Check sheet for the modelled part. Datum: model origin and axes. Units: mm. A direction names the side the tool comes from. Give positions to 0.01 mm unless a question says otherwise; leave off trailing zeros. Loops run counter-clockwise (first coordinate to the right, second up) from the corner with the lowest first, then second, coordinate; pieces in that order, holes last. Notation, with made-up numbers: (-18, 18.5) -> (-5, 18.5) arc R15 cw to (-5, 42.5) -> close; hole circle Ø10 at (-30, 89.25). An arc over 180 degrees is marked (long way). Answer as CSV lines item,"result". Start each with the question number.
(1) Gauge pin test, flat ends, axial feed: pin 1 Ø0.8 at (x, y) = (-133, 20) entering from +Z (3 decimals); pin 2 Ø9.5 at (x, y) = (15, 28.5) entering from -Z; pin 3 Ø1.3 at (y, z) = (12.5, -132.5) entering from +X (3 decimals). Record the tip position at first contact, or that the pin passes through.
(2) Access from +Z, -Z, +X, -X, +Y, -Y to the whole of each face (thin tool, end or side, straight path). Record for faces 5 (the face through (-59.797, 5.027, -62.042)), 6 (the face through (35, 19, -131.724)), 7 (the face through (-85.2, 18.46, -85.23)).
(3) Material ranges on line 1 (Y direction, x = -53, z = -52) (3 decimals); line 2 (X direction, y = 6, z = -23.5) (3 decimals); line 3 (Z direction, x = -102, y = 2) (3 decimals), recorded low to high. Write a range as from..to.
(4) Section check B-B on x = -49.5. Enter the section's corners in (y, z) (3 decimals), plus the area to 3 significant figures.
(5) Section check A-A on z = -82. Enter the section's corners in (x, y) (3 decimals), plus the area to 3 significant figures.
(6) Release check for a two-part mould opening along Y. For faces 1 (the face through (-97, 11.176, -89)), 2 (the face through (36.908, 6.437, -130.973)), 3 (the face through (-45, 0, -46)), 4 (the face through (0, 4, -86)) record: pulls with the +Y half, pulls with the -Y half, needs draft (parallel to the pull), parting line crosses it, or undercut.
(7) Section check C-C on z = -119. Enter the section's corners in (x, y) (3 decimals), plus the area to 3 significant figures.
from build123d import *

# Parameters (mm, degrees)
SKETCH1_R            = 15
BOSS_EXTRUDE2_DEPTH  = 8.255
BOSS_EXTRUDE3_DEPTH  = 8.255
BOSS_EXTRUDE4_DEPTH  = 38.1
SKETCH5_R            = 3.249999977
CUT_EXTRUDE3_DEPTH   = 63.5
BOSS_EXTRUDE9_DEPTH  = 3.175
BOSS_EXTRUDE11_DEPTH = 3.175
BOSS_EXTRUDE14_DEPTH = 3.175
SKETCH15_W           = 38.1
SKETCH15_H           = 44.45
BOSS_EXTRUDE15_DEPTH = 1.524
SKETCH16_W           = 38.1
SKETCH16_H           = 44.45
BOSS_EXTRUDE16_DEPTH = 1.524
SKETCH17_R           = 1.98501
CUT_EXTRUDE4_DEPTH   = 2.54
SKETCH18_R           = 1.98501
CUT_EXTRUDE5_DEPTH   = 2.54
SKETCH19_W           = 19.05
SKETCH19_H           = 38.1
BOSS_EXTRUDE17_DEPTH = 1.587961
SKETCH20_W           = 19.05
SKETCH20_H           = 38.1
BOSS_EXTRUDE18_DEPTH = 1.587961
CUT_EXTRUDE6_REACH   = 202.702
SKETCH21_R           = 1.524
BOSS_EXTRUDE20_START = -0.60614
SKETCH21_3_W         = 25.4
SKETCH21_3_H         = 22.86
SKETCH21_3_R         = 1.524
BOSS_EXTRUDE20_DEPTH = 0.60614
CUT_EXTRUDE7_REACH   = 202.702
SKETCH26_W           = 6.858
SKETCH26_H           = 5.334


with BuildPart() as part:
    # Sketch1 → Boss-Extrude2 (new body)
    with BuildSketch(Plane(origin=(0, 0, 0), x_dir=(1, 0, 0), z_dir=(0, 1, 0))):
        Circle(SKETCH1_R)
    extrude(amount=BOSS_EXTRUDE2_DEPTH)

    # Sketch1<6> → Boss-Extrude3 (add)
    with BuildSketch(Plane(origin=(0, 0, 0), x_dir=(1, 0, 0), z_dir=(0, 1, 0))):
        with BuildLine():
            ThreePointArc((3.175, 130.136274728), (1.587618078, 130.165318322), (0, 130.175))
            Line((0, 130.175), (0, 15))
            ThreePointArc((0, 15), (1.596569562, 14.914790164), (3.175, 14.660128751))
            Line((3.175, 14.660128751), (3.175, 130.136274728))
        make_face()
        with BuildLine():
            Line((-9.42450178, 11.66956581), (-90.918248264, 93.163312294))
            ThreePointArc((-90.918248264, 93.163312294), (-92.047625241, 92.047625241), (-93.163312294, 90.918248264))
            Line((-93.163312294, 90.918248264), (-11.66956581, 9.42450178))
            ThreePointArc((-11.66956581, 9.42450178), (-10.606601718, 10.606601718), (-9.42450178, 11.66956581))
        make_face()
        with BuildLine():
            Line((-15, 0), (-130.175, 0))
            ThreePointArc((-130.175, 0), (-130.165318322, -1.587618078), (-130.136274728, -3.175))
            Line((-130.136274728, -3.175), (-14.660128751, -3.175))
            ThreePointArc((-14.660128751, -3.175), (-14.914790164, -1.596569562), (-15, 0))
        make_face()
    extrude(amount=BOSS_EXTRUDE3_DEPTH)

    # Sketch1<7> → Boss-Extrude4 (add)
    with BuildSketch(Plane(origin=(0, 0, 0), x_dir=(1, 0, 0), z_dir=(0, 1, 0))):
        with BuildLine():
            Line((3.175, 130.136274728), (3.175, 133.312197023))
            ThreePointArc((3.175, 133.312197023), (-94.292689271, 94.292689271), (-133.312197023, -3.175))
            Line((-133.312197023, -3.175), (-130.136274728, -3.175))
            ThreePointArc((-130.136274728, -3.175), (-92.047625241, 92.047625241), (3.175, 130.136274728))
        make_face()
    extrude(amount=BOSS_EXTRUDE4_DEPTH)

    # Sketch5 → Cut-Extrude3 (cut)
    with BuildSketch(Plane(origin=(0, 8.255, 0), x_dir=(1, 0, 0), z_dir=(0, 1, 0))):
        Circle(SKETCH5_R)
        with BuildLine():
            Line((-7.236078848, 3.458556767), (-9.686234559, 5.271576621))
            ThreePointArc((-9.686234559, 5.271576621), (-10.004802487, 7.403164404), (-7.873214705, 7.721732332))
            Line((-7.873214705, 7.721732332), (-5.423058993, 5.908712478))
            ThreePointArc((-5.423058993, 5.908712478), (-5.104491065, 3.777124696), (-7.236078848, 3.458556767))
        make_face()
        with BuildLine():
            Line((5.423058993, -5.908712478), (7.873214705, -7.721732332))
            ThreePointArc((7.873214705, -7.721732332), (10.004802487, -7.403164404), (9.686234559, -5.271576621))
            Line((9.686234559, -5.271576621), (7.236078848, -3.458556767))
            ThreePointArc((7.236078848, -3.458556767), (5.104491065, -3.777124696), (5.423058993, -5.908712478))
        make_face()
    extrude(amount=-CUT_EXTRUDE3_DEPTH, mode=Mode.SUBTRACT)

    # Sketch10 → Boss-Extrude9 (add)
    with BuildSketch(Plane(origin=(0, 0, 0), x_dir=(-1, 0, 0), z_dir=(0, 0, -1))):
        Polygon((130.175, 27.305), (130.175, 8.255), (111.125, 8.255), align=None)
    extrude(amount=-BOSS_EXTRUDE9_DEPTH)

    # Sketch13 → Boss-Extrude11 (add)
    with BuildSketch(Plane.ZY):
        Polygon((-130.175, 27.305), (-111.125, 8.255), (-130.175, 8.255), align=None)
    extrude(amount=-BOSS_EXTRUDE11_DEPTH)

    # Sketch14 → Boss-Extrude14 (add)
    with BuildSketch(Plane(origin=(1.122532015, 0, -1.122532015), x_dir=(-0.707106781, 0, -0.707106781), z_dir=(0.707106781, 0, -0.707106781))):
        Polygon((133.340319762, 8.255), (111.115319762, 8.255), (133.340319762, 32.394680238), align=None)
    extrude(amount=-BOSS_EXTRUDE14_DEPTH)

    # Sketch15 → Boss-Extrude15 (add)
    with BuildSketch(Plane(origin=(-131.724235875, 0, 0), x_dir=(0, -1, 0), z_dir=(-1, 0, 0))):
        with Locations((-19.05, 25.4)):
            Rectangle(SKETCH15_W, SKETCH15_H)
    extrude(amount=-BOSS_EXTRUDE15_DEPTH)

    # Sketch16 → Boss-Extrude16 (add)
    with BuildSketch(Plane(origin=(0, 0, -131.724235875), x_dir=(0, -1, 0), z_dir=(0, 0, -1))):
        with Locations((-19.05, -25.4)):
            Rectangle(SKETCH16_W, SKETCH16_H)
    extrude(amount=-BOSS_EXTRUDE16_DEPTH)

    # Sketch17 → Cut-Extrude4 (cut)
    with BuildSketch(Plane(origin=(0, 0, -131.724235875), x_dir=(-1, 0, 0), z_dir=(0, 0, -1))):
        with Locations((-34.925, 31.75)):
            Circle(SKETCH17_R)
        with Locations((-34.925, 6.35)):
            Circle(SKETCH17_R)
    extrude(amount=-CUT_EXTRUDE4_DEPTH, mode=Mode.SUBTRACT)

    # Sketch18 → Cut-Extrude5 (cut)
    with BuildSketch(Plane.ZY.offset(131.724235875)):
        with Locations((34.925, 31.75)):
            Circle(SKETCH18_R)
        with Locations((34.925, 6.35)):
            Circle(SKETCH18_R)
    extrude(amount=-CUT_EXTRUDE5_DEPTH, mode=Mode.SUBTRACT)

    # Sketch19 → Boss-Extrude17 (add)
    with BuildSketch(Plane.ZY.offset(131.724235875)):
        with Locations((12.7, 19.05)):
            Rectangle(SKETCH19_W, SKETCH19_H)
    extrude(amount=BOSS_EXTRUDE17_DEPTH)

    # Sketch20 → Boss-Extrude18 (add)
    with BuildSketch(Plane(origin=(0, 0, -131.724235875), x_dir=(-1, 0, 0), z_dir=(0, 0, -1))):
        with Locations((-12.7, 19.05)):
            Rectangle(SKETCH20_W, SKETCH20_H)
    extrude(amount=BOSS_EXTRUDE18_DEPTH)

    # Sketch21 → Cut-Extrude6 (cut, up to next)
    with BuildSketch(Plane(origin=(-94.292689271, 0, -94.292689271), x_dir=(-0.707106781, 0, 0.707106781), z_dir=(-0.707106781, 0, -0.707106781)), mode=Mode.PRIVATE) as cut_extrude6_sk1:
        with Locations((8.636, 4.064)):
            Circle(SKETCH21_R)
    cut_extrude6_tool1 = extrude(cut_extrude6_sk1.sketch, amount=-CUT_EXTRUDE6_REACH, mode=Mode.PRIVATE) & part.part
    add(cut_extrude6_tool1.solids().sort_by_distance((-100.399263, 4.064, -88.186115))[0], mode=Mode.SUBTRACT)
    # Sketch21 → Cut-Extrude6 (cut, up to next)
    with BuildSketch(Plane(origin=(-94.292689271, 0, -94.292689271), x_dir=(-0.707106781, 0, 0.707106781), z_dir=(-0.707106781, 0, -0.707106781)), mode=Mode.PRIVATE) as cut_extrude6_sk2:
        with Locations((-8.636, 18.796)):
            Circle(SKETCH21_R)
    cut_extrude6_tool2 = extrude(cut_extrude6_sk2.sketch, amount=-CUT_EXTRUDE6_REACH, mode=Mode.PRIVATE) & part.part
    add(cut_extrude6_tool2.solids().sort_by_distance((-88.186115, 18.796, -100.399263))[0], mode=Mode.SUBTRACT)

    # Sketch21<3> → Boss-Extrude20 (add)
    with BuildSketch(Plane(origin=(-94.292689271, 0, -94.292689271), x_dir=(-0.707106781, 0, 0.707106781), z_dir=(-0.707106781, 0, -0.707106781)).offset(BOSS_EXTRUDE20_START)):
        with Locations((0, 11.43)):
            Rectangle(SKETCH21_3_W, SKETCH21_3_H)
        with Locations((8.636, 4.064)):
            Circle(SKETCH21_3_R, mode=Mode.SUBTRACT)
        with Locations((-8.636, 18.796)):
            Circle(SKETCH21_3_R, mode=Mode.SUBTRACT)
    extrude(amount=BOSS_EXTRUDE20_DEPTH)

    # Sketch26 → Cut-Extrude7 (cut, up to next)
    with BuildSketch(Plane(origin=(-94.292689271, 0, -94.292689271), x_dir=(-0.707106781, 0, 0.707106781), z_dir=(-0.707106781, 0, -0.707106781)), mode=Mode.PRIVATE) as cut_extrude7_sk1:
        with Locations((6.096, 13.843)):
            Rectangle(SKETCH26_W, SKETCH26_H)
    cut_extrude7_tool1 = extrude(cut_extrude7_sk1.sketch, amount=-CUT_EXTRUDE7_REACH, mode=Mode.PRIVATE) & part.part
    add(cut_extrude7_tool1.solids().sort_by_distance((-98.603212, 13.843, -89.982166))[0], mode=Mode.SUBTRACT)


solid = part.part
Working result:
1,pin 1,"stops at z = 22.225"
1,pin 2,"stops at z = -133.31"
1,pin 3,"stops at x = 22.225"
2,face 5,"+Y, -Y"
2,face 6,"-Z, +X, +Y, -Y"
2,face 7,"+Z, +X, +Y"
3,line 1,"y = 0..8.255"
3,line 2,"x = -131.263..-128.036, -25.745..-21.255, 0..3.175"
3,line 3,"z = -86.585..-80.88, 0..3.175"
4,outline,"(0, -123.822) -> (38.1, -123.822) -> (38.1, -120.396) -> (0, -120.396) -> close; (0, -51.745) -> (8.255, -51.745) -> (8.255, -47.255) -> (0, -47.255) -> close; (0, 0) -> (8.255, 0) -> (8.255, 3.175) -> (0, 3.175) -> close"
4,area,"194 mm^2"
5,outline,"(-105.158, 0) -> (-101.102, 0) -> (-101.102, 38.1) -> (-105.158, 38.1) -> close; (-84.245, 0) -> (-79.755, 0) -> (-79.755, 11.799) -> (-84.245, 15.247) -> close; (0, 0) -> (3.175, 0) -> (3.175, 8.255) -> (0, 8.255) -> close"
5,area,"241 mm^2"
6,face 1,"undercut"
6,face 2,"undercut"
6,face 3,"pulls with the -Y half"
6,face 4,"needs draft"
7,outline,"(-60.177, 0) -> (-52.769, 0) -> (-52.769, 38.1) -> (-60.177, 38.1) -> close; (0, 0) -> (3.175, 0) -> (3.175, 16.13) -> (0, 16.13) -> close"
7,area,"333 mm^2"
